Input: part model. Units: mm. Frame: model coordinates. A direction names the side the tool comes from. Round coordinates to 2 decimals unless told otherwise and drop trailing zeros. Loops run counter-clockwise (first coordinate to the right, second up) from the corner with the lowest first, then second, coordinate; pieces in that order, holes last. Notation, with made-up numbers: M -1.75,-35 L 14.25,-35 A17 ccw 14.25,-7 Z; hole C -20,65 d7. An arc over 180 degrees is marked long. Use one line per item in the form item = value. Start each with the question number.
Q1. Section query B-B, the plane z = -10. Output: boundary loops of the cut face in (x, y).
Q2. Access query for faces 5 (the flat face through (0, 8, -2.165)), 6 (the flat face through (9.822, 8, -1)), 7 (the flat face through (52.209, 1, -10)). Directions: +Z, -Z, +X, -X, +Y, -Y. A direction counts if a zero-diameter tool reaches every point of the face in a straight line with its end or side. Return the directions, or none.
Q3. Section query A-A, the plane y = 9.25. Output: boundary loops of the cut face in (x, z), and give its area (3 significant figures).
Q4. Mould query, pull axis X, two halves, no side actions, for faces 1 (the flat face through (-1, 3, -10)), 2 (the cylindrical face through (2.969, 10.985, -1.151)), 3 (the flat face through (-10.178, 8, -1)), 4 (the cylindrical face through (-4.843, 10.433, -1.151)). Classes: pulls with the +X half, pulls with the -X half, needs draft (parallel to the pull), parting line crosses it, or undercut.
Q5. Ray query, line 1 along Y through (x, z) = (18, -7.25); line 2 along X through (y, z) = (6, -2); line 3 along Z through (x, y) = (7, 11.75). Return the intervals inside material, ascending.
Q6. Section query C-C, the plane x = 21.5. Output: boundary loops of the cut face in (y, z), and give its area (3 significant figures).
Q7. First-contact query: P1, Ø1, axis at y = 8.5, z = -1.5, coming from the +X side; P2, Ø0.6, axis at y = 9, z = -1.5, coming from the -X side; P3, Ø6, axis at x = -25, z = -10, coming from the +Y side. Flat tips, straight axial feed; report the tip coordinate or a pass-through.
```python
from build123d import *

# Parameters (mm, degrees)
ESQUISSE1_W             = 104
ESQUISSE1_H             = 20
ESQUISSE1_R             = 2.1
BOSS_EXTRU_1_DEPTH      = 3
BOSS_EXTRU_2_DEPTH      = 10
ESQUISSE3_R             = 1.75
ENL_V_MAT_EXTRU_1_DEPTH = 10


with BuildPart() as part:
    # Esquisse1 → Boss.-Extru.1 (new body)
    with BuildSketch(Plane(origin=(0, 0, 0), x_dir=(1, 0, 0), z_dir=(0, 1, 0))):
        with Locations((0.208658176, 10.165016502)):
            Rectangle(ESQUISSE1_W, ESQUISSE1_H)
        with Locations(Location((-43.791341824, 10.165016502, 0), (0, 0, 270))):
            Circle(ESQUISSE1_R, mode=Mode.SUBTRACT)
        with Locations(Location((44.208658176, 10.165016502, 0), (0, 0, 270))):
            Circle(ESQUISSE1_R, mode=Mode.SUBTRACT)
    extrude(amount=BOSS_EXTRU_1_DEPTH)

    # Esquisse2 → Boss.-Extru.2 (add)
    with BuildSketch(Plane(origin=(0, 3, 0), x_dir=(1, 0, 0), z_dir=(0, 1, 0))):
        Polygon((-0.177943938, 0.165016502), (-10.177943938, 0.165016502), (-10.177943938, 2.165016502), (9.822056062, 2.165016502), (9.822056062, 0.165016502), align=None)
    extrude(amount=BOSS_EXTRU_2_DEPTH)

    # Esquisse3 → Enlèv. mat.-Extru.1 (cut)
    with BuildSketch(Plane.XY.offset(-0.165016502)):
        with Locations((-3.552943938, 9.25)):
            Circle(ESQUISSE3_R)
        with Locations((3.197056062, 9.25)):
            Circle(ESQUISSE3_R)
    extrude(amount=-ENL_V_MAT_EXTRU_1_DEPTH, mode=Mode.SUBTRACT)


solid = part.part
```
Results found:
q1.outline = M -51.79,0 L -45.88,0 L -45.88,3 L -51.79,3 Z; M -41.7,0 L 42.12,0 L 42.12,3 L -41.7,3 Z; M 46.3,0 L 52.21,0 L 52.21,3 L 46.3,3 Z
q2.face_5 = -Z, +X, -X, +Y
q2.face_6 = +Z, -Z, +X, +Y
q2.face_7 = +Z, -Z, +X, +Y, -Y
q3.outline = M -10.18,-2.17 L -5.3,-2.17 L -5.3,-0.17 L -10.18,-0.17 Z; M -1.8,-2.17 L 1.45,-2.17 L 1.45,-0.17 L -1.8,-0.17 Z; M 4.95,-2.17 L 9.82,-2.17 L 9.82,-0.17 L 4.95,-0.17 Z
q3.area = 26.0 mm²
q4.face_1 = needs draft
q4.face_2 = undercut
q4.face_3 = pulls with the -X half
q4.face_4 = undercut
q5.line_1 = 0 to 3
q5.line_2 = -10.18 to 9.82
q5.line_3 = -2.17 to -0.17
q6.outline = M 0,-20.17 L 3,-20.17 L 3,-0.17 L 0,-0.17 Z
q6.area = 60.0 mm²
q7.P1 = 9.82
q7.P2 = -10.18
q7.P3 = 3
